Read the model definition and answer for the solid it produces. Units are mm, in the model's axes. A direction names the side the tool comes from. Coordinates: 2 decimals unless noted, no trailing zeros. Order: outer loops, then holes, each group sorted by start corner. A loop starts at its lowest first (then second) coordinate and runs counter-clockwise, first axis right, second up. Notation, with made-up numbers: (1.5, 34.5) -> (53.5, 34.5) arc R19 ccw to (53.5, 55.5) -> close; hole circle Ø4 at (47, -4.5). An arc over 180 degrees is marked (long way). Return JSON: item names as keys, results as strings. Group by question number.
```python
from build123d import *

# Parameters (mm, degrees)
SKETCH2_W                      = 1841.5
SKETCH2_H                      = 69.6722
BASE_FLANGE1_DEPTH             = 3.2639
EDGE_FLANGE1_STRIP_W           = 15.5956
EDGE_FLANGE1_STRIP_H           = 3.2639
EDGE_FLANGE1_STRIP_CUT_DEPTH   = 1841.5
EDGE_FLANGE1_STRIP_2_W         = 15.5956
EDGE_FLANGE1_STRIP_2_H         = 3.2639
EDGE_FLANGE1_STRIP_CUT_2_DEPTH = 1841.5
EDGE_FLANGE1_DEPTH             = 1841.5
EDGE_FLANGE1_BEND_DEPTH        = 1841.5
F_10_0_1935_DIAMETER_HOLE1_D   = 4.9149
F_10_0_1935_DIAMETER_HOLE3_D   = 4.9149
F_10_0_1935_DIAMETER_HOLE4_D   = 4.9149
F_10_0_2_DIAMETER_HOLE1_D      = 5.08
F_10_0_1935_DIAMETER_HOLE6_D   = 4.9149
LPATTERN2_COUNT                = 3
LPATTERN2_PITCH                = 381
CUT_EXTRUDE1_DEPTH             = 926.779934253
FILLET2_R                      = 6.35


# Sheet-metal steps are written as plain solids
with BuildPart() as part:
    # Sketch2 → Base-Flange1 (new body)
    with BuildSketch(Plane.XY):
        Rectangle(SKETCH2_W, SKETCH2_H)
    extrude(amount=-BASE_FLANGE1_DEPTH)

    # Edge-Flange1 strip (across the edge) → Edge-Flange1 strip cut (cut)
    with BuildSketch(Plane(origin=(920.75, 34.8361, 0), x_dir=(0, -1, 0), z_dir=(-1, 0, 0))):
        with Locations((-3.2639, -1.63195)):
            Rectangle(EDGE_FLANGE1_STRIP_W, EDGE_FLANGE1_STRIP_H)
    extrude(amount=EDGE_FLANGE1_STRIP_CUT_DEPTH, mode=Mode.SUBTRACT)

    # Edge-Flange1 strip 2 (across the edge) → Edge-Flange1 strip cut 2 (cut)
    with BuildSketch(Plane(origin=(-920.75, -34.8361, 0), x_dir=(0, 1, 0), z_dir=(1, 0, 0))):
        with Locations((-3.2639, -1.63195)):
            Rectangle(EDGE_FLANGE1_STRIP_2_W, EDGE_FLANGE1_STRIP_2_H)
    extrude(amount=EDGE_FLANGE1_STRIP_CUT_2_DEPTH, mode=Mode.SUBTRACT)

    # Edge-Flange1 section (across the edge) → Edge-Flange1 (add)
    with BuildSketch(Plane(origin=(920.75, 34.8361, 0), x_dir=(0, -1, 0), z_dir=(-1, 0, 0))):
        with BuildLine():
            Line((0, 1.27), (0, 66.5861))
            Line((0, 66.5861), (3.2639, 66.5861))
            Line((3.2639, 66.5861), (3.2639, 1.27))
            ThreePointArc((3.2639, 1.27), (3.635874388, 0.371974388), (4.5339, 0))
            Line((4.5339, 0), (4.5339, -3.2639))
            ThreePointArc((4.5339, -3.2639), (1.327948565, -1.935951435), (0, 1.27))
        make_face()
    extrude(amount=EDGE_FLANGE1_DEPTH)

    # Edge-Flange1 section 2 (across the edge) → Edge-Flange1 bend (add)
    with BuildSketch(Plane(origin=(-920.75, -34.8361, 0), x_dir=(0, 1, 0), z_dir=(1, 0, 0))):
        with BuildLine():
            Line((0, 1.27), (0, 66.5861))
            Line((0, 66.5861), (3.2639, 66.5861))
            Line((3.2639, 66.5861), (3.2639, 1.27))
            ThreePointArc((3.2639, 1.27), (3.635874388, 0.371974388), (4.5339, 0))
            Line((4.5339, 0), (4.5339, -3.2639))
            ThreePointArc((4.5339, -3.2639), (1.327948565, -1.935951435), (0, 1.27))
        make_face()
    extrude(amount=EDGE_FLANGE1_BEND_DEPTH)

    # #10 (0.1935) Diameter Hole1 (through all)
    with Locations(Plane(origin=(0, 34.8361, 34.8361), x_dir=(-1, 0, 0), z_dir=(0, 1, 0))):
        with Locations((800.1, -23.13305), (800.1, 21.31695), (850.9, 21.31695), (850.9, -23.13305), (901.7, 21.31695), (901.7, -23.13305)):
            Hole(F_10_0_1935_DIAMETER_HOLE1_D / 2)

    # #10 (0.1935) Diameter Hole3 (through all)
    with Locations(Plane(origin=(0, 34.8361, 0), x_dir=(1, 0, 0), z_dir=(0, 1, 0))):
        with Locations((819.15, -14.87805), (819.15, -52.97805), (895.35, -14.87805), (895.35, -52.97805)):
            Hole(F_10_0_1935_DIAMETER_HOLE3_D / 2)

    # #10 (0.1935) Diameter Hole4 (through all)
    with Locations(Plane(origin=(0, 34.8361, 0), x_dir=(1, 0, 0), z_dir=(0, 1, 0))):
        with Locations((520.7, -14.87805), (558.8, -14.87805), (558.8, -52.97805), (520.7, -52.97805)):
            Hole(F_10_0_1935_DIAMETER_HOLE4_D / 2)

    # #10 (0.2) Diameter Hole1 (through all)
    with Locations(Plane(origin=(0, 34.8361, 0), x_dir=(1, 0, 0), z_dir=(0, 1, 0))):
        with Locations((-761.32055, -33.92805), (-678.77055, -33.92805)):
            Hole(F_10_0_2_DIAMETER_HOLE1_D / 2)

    # #10 (0.1935) Diameter Hole6 (through all)
    with Locations(Plane(origin=(0, -34.8361, 0), x_dir=(-1, 0, 0), z_dir=(0, -1, 0))):
        with Locations((463.55, -10.795)):
            f_10_0_1935_diameter_hole6 = Hole(F_10_0_1935_DIAMETER_HOLE6_D / 2)

    # LPattern2: #10 (0.1935) Diameter Hole6 ×3
    with Locations(*[(i * LPATTERN2_PITCH, 0, 0) for i in range(1, LPATTERN2_COUNT)]):
        add(f_10_0_1935_diameter_hole6, mode=Mode.SUBTRACT)

    # Sketch46 → Cut-Extrude1 (cut, through all)
    with BuildSketch(Plane(origin=(0, 34.8361, 0), x_dir=(1, 0, 0), z_dir=(0, 1, 0))):
        Polygon((-641.35, -28.4861), (-641.35, -66.5861), (476.25, -66.5861), (476.25, -28.4861), (-82.55, -28.4861), align=None)
    extrude(amount=-CUT_EXTRUDE1_DEPTH, mode=Mode.SUBTRACT)

    # Fillet2
    fillet2_edges = [part.edges().sort_by_distance(p)[0] for p in [
        (476.25, 33.20415, 66.5861),
        (-641.35, 33.20415, 28.4861),
        (-641.35, 33.20415, 66.5861),
        (476.25, 33.20415, 28.4861),
        (476.25, -33.20415, 66.5861),
        (-641.35, -33.20415, 66.5861),
        (-641.35, -33.20415, 28.4861),
        (476.25, -33.20415, 28.4861),
        (920.75, 33.20415, 66.5861),
        (-920.75, 33.20415, 66.5861),
        (-920.75, -33.20415, 66.5861),
        (920.75, -33.20415, 66.5861),
    ]]
    fillet(fillet2_edges, radius=FILLET2_R)


solid = part.part
```
1. Find section A-A on x = -226. Determine the outline of the cut face in (y, z), and give its area (3 significant figures).
2. Straight lines are drawn through the part: L1, parallel to Z at x = 819, y = -32; L2, parallel to Y at x = 184, z = 20; L3, parallel to Z at x = 831.5, y = -9. For each, find the intervals that lie inside material, in ascending order.
3. Which of the six approach directions +Z, -Z, +X, -X, +Y, -Y give full straight-line access (tool end or side, diameter ignored) to faces 5 (the face through (-13, 0, -3.264)), 6 (the face through (13, 31.572, 27))?
4. Given pin 1 (3.5 mm diameter, centred on x = 13.5, y = 33.5, fed in from +Z); pin 2 (6 mm diameter, centred on x = 179, y = -17.5, fed in from +Z), each flat-ended and moving along its own axis, determine where each tip first touches the part or whether it passes through.
5. Find section B-B on y = 4.5. Determine the outline of the cut face in (x, z).
6. Find section C-C on x = 676. Determine the outline of the cut face in (y, z).
7. For a pull along Y with two mould halves and no side action, classify faces 1 (the face through (-13, 0, 0)), 2 (the face through (920.75, 0, -2)), 3 (the face through (-13, -34.836, 26)), 4 (the face through (13, 34.836, 26)) as released by +Y, released by -Y, zero draft, split by the parting line, or undercut.
Result:
{
 "1": {"outline": "(-34.84, 1.27) arc R4.53 ccw to (-30.3, -3.26) -> (30.3, -3.26) arc R4.53 ccw to (34.84, 1.27) -> (34.84, 28.49) -> (31.57, 28.49) -> (31.57, 1.27) arc R1.27 cw to (30.3, 0) -> (-30.3, 0) arc R1.27 cw to (-31.57, 1.27) -> (-31.57, 28.49) -> (-34.84, 28.49) -> close", "area": "405 mm^2"},
 "2": {"L1": "-2.93 to 12.43, 17.33 to 50.53, 55.43 to 66.59", "L2": "-34.84 to -31.57, 31.57 to 34.84", "L3": "-3.26 to 0"},
 "3": {"face 5": "-Z, +X, -X, +Y, -Y", "face 6": "+Z, +X, -X"},
 "4": {"pin 1": "z = 28.49", "pin 2": "z = 0"},
 "5": {"outline": "(-920.75, -3.26) -> (920.75, -3.26) -> (920.75, 0) -> (-920.75, 0) -> close"},
 "6": {"outline": "(-34.84, 1.27) arc R4.53 ccw to (-30.3, -3.26) -> (30.3, -3.26) arc R4.53 ccw to (34.84, 1.27) -> (34.84, 66.59) -> (31.57, 66.59) -> (31.57, 1.27) arc R1.27 cw to (30.3, 0) -> (-30.3, 0) arc R1.27 cw to (-31.57, 1.27) -> (-31.57, 66.59) -> (-34.84, 66.59) -> close"},
 "7": {"face 1": "undercut", "face 2": "zero draft", "face 3": "released by -Y", "face 4": "released by +Y"}
}
